from build123d import *

# Parameters (mm, degrees)
SKETCH1_W           = 20
SKETCH1_H           = 20
SKETCH1_R           = 1
BOSS_EXTRUDE1_DEPTH = 4
SKETCH2_W           = 20
SKETCH2_H           = 40
SKETCH2_R           = 3
BOSS_EXTRUDE2_DEPTH = 4
FILLET1_R           = 5
SKETCH3_R           = 3
BOSS_EXTRUDE3_DEPTH = 20


with BuildPart() as part:
    # Sketch1 → Boss-Extrude1 (new body)
    with BuildSketch(Plane(origin=(0, 0, 0), x_dir=(1, 0, 0), z_dir=(0, 1, 0))):
        Rectangle(SKETCH1_W, SKETCH1_H)
        with Locations(Location((-8, 8, 0), (0, 0, 270))):
            Circle(SKETCH1_R, mode=Mode.SUBTRACT)
        with Locations(Location((-8, -8, 0), (0, 0, 270))):
            Circle(SKETCH1_R, mode=Mode.SUBTRACT)
        with Locations(Location((8, -8, 0), (0, 0, 270))):
            Circle(SKETCH1_R, mode=Mode.SUBTRACT)
        with Locations(Location((8, 8, 0), (0, 0, 270))):
            Circle(SKETCH1_R, mode=Mode.SUBTRACT)
    extrude(amount=BOSS_EXTRUDE1_DEPTH)

    # Sketch2 → Boss-Extrude2 (add)
    with BuildSketch(Plane(origin=(0, 0, -10), x_dir=(-1, 0, 0), z_dir=(0, 0, -1))):
        with Locations((0, 20)):
            Rectangle(SKETCH2_W, SKETCH2_H)
        with Locations((0, 25)):
            Circle(SKETCH2_R, mode=Mode.SUBTRACT)
    extrude(amount=BOSS_EXTRUDE2_DEPTH)

    # Fillet1
    fillet1_edges = [part.edges().sort_by_distance(p)[0] for p in [
        (0, 0, -14),
    ]]
    fillet(fillet1_edges, radius=FILLET1_R - 0.0001)  # a hair under: the kernel refuses the full size

    # Sketch3 → Boss-Extrude3 (add)
    with BuildSketch(Plane.XY.offset(-10)):
        with Locations((0, 25)):
            Circle(SKETCH3_R)
    extrude(amount=-BOSS_EXTRUDE3_DEPTH)


solid = part.part
Geometry check sheet. Reference: the model listing, model coordinates, mm. A direction names the side the tool comes from. Coordinates: 2 decimals unless noted, no trailing zeros. Order: outer loops, then holes, each group sorted by start corner. A loop starts at its lowest first (then second) coordinate and runs counter-clockwise, first axis right, second up. Notation, with made-up numbers: (86, 23.25) - (132, 23.25) arc R27 cw to (132, 58.25) - close; hole circle Ø10 at (-16, -15). An arc over 180 degrees is marked (long way). Answer in a Markdown table with one row per item. Add a question column.
1) Cross-section at C-C, the plane y = 25. Record the cut outline in (x, z), then the cut area to 3 significant figures.
2) Cross-section at A-A, the plane x = 8. State how many separate pieces and enclosed holes the cut face has, then the cut area to 3 significant figures.
3) Cross-section at D-D, the plane x = 0. Record the cut outline in (y, z).
4) Set-up check for faces 1 (the cylindrical face through (9, 2, 8)), 2 (the flat face through (0, 4, 0)), 3 (the cylindrical face through (-0.65, 22.07, -21.89)): record each of +Z, -Z, +X, -X, +Y, -Y from which the full face is reachable in a straight line by a thin tool's end or side.
5) Cross-section at B-B, the plane z = 8. Record the cut outline in (x, y), then the cut area to 3 significant figures.
6) Material ranges on line 1 along X through (y, z) = (2.95, 8); line 2 along Z through (x, y) = (7.5, 15); line 3 along Y through (x, z) = (3.5, -1), recorded low to high. Write a range as [from, to].
7) Release check for a two-part mould opening along Z. For faces 4 (the flat face through (2.4, 22.7, -14)), 5 (the flat face through (0, 22, -10)), 6 (the cylindrical face through (9, 2, -8)), 7 (the flat face through (0, 40, -12)) record: +Z half, -Z half, draft (parallel to the pull), parting line (faces both ways), or undercut.
8) Gauge pin test, flat ends, axial feed: P1, Ø2, axis at x = 2, y = 35.5, coming from the +Z side; P2, Ø5, axis at x = -6, y = 24, coming from the -Z side; P3, Ø1.6, axis at x = -8, z = -8, coming from the -Y side; P4, Ø10, axis at x = -0.5, z = -22.5, coming from the -Y side. Record the tip position at first contact, or that the pin passes through.
Check result:
| question | item | result |
|---|---|---|
| 1 | outline | (-10, -14) - (-3, -14) - (-3, -30) - (3, -30) - (3, -14) - (10, -14) - (10, -10) - (-10, -10) - close |
| 1 | area | 176 mm² |
| 2 | separate pieces | 3 |
| 2 | enclosed holes | 0 |
| 2 | area | 219 mm² |
| 3 | outline | (0, -9) arc R5 ccw to (5, -14) - (22, -14) - (22, -30) - (28, -30) - (28, -14) - (40, -14) - (40, -10) - (4, -10) - (4, 10) - (0, 10) - close |
| 4 | face 1 | +Y, -Y |
| 4 | face 2 | +Z, +X, -X, +Y |
| 4 | face 3 | -Z |
| 5 | outline | (-10, 0) - (-9, 0) - (-9, 4) - (-10, 4) - close; (-7, 0) - (7, 0) - (7, 4) - (-7, 4) - close; (9, 0) - (10, 0) - (10, 4) - (9, 4) - close |
| 5 | area | 64.0 mm² |
| 6 | line 1 | x = [-10, -9], [-7, 7], [9, 10] |
| 6 | line 2 | z = [-14, -10] |
| 6 | line 3 | y = [0, 4] |
| 7 | face 4 | -Z half |
| 7 | face 5 | +Z half |
| 7 | face 6 | undercut |
| 7 | face 7 | draft |
| 8 | P1 | stops at z = -10 |
| 8 | P2 | stops at z = -14 |
| 8 | P3 | passes through |
| 8 | P4 | stops at y = 22 |
